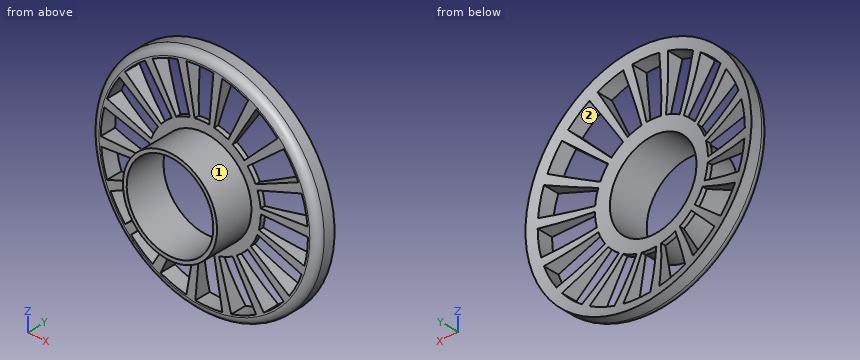
```python
from build123d import *

# Parameters (mm, degrees)
SKETCH1_R           = 12.5
BOSS_EXTRUDE1_DEPTH = 10
SKETCH3_R           = 30
BOSS_EXTRUDE2_DEPTH = 5
DOME1_FACE_RADIUS   = 30
DOME1_HEIGHT        = 5
SKETCH8_R           = 11.5
CUT_EXTRUDE3_DEPTH  = 46
CUT_EXTRUDE4_DEPTH  = 44.588989435
FILLET2_R           = 2


with BuildPart() as part:
    # Sketch1 → Boss-Extrude1 (new body)
    with BuildSketch(Plane(origin=(0, 0, 0), x_dir=(1, 0, 0), z_dir=(0, 1, 0))):
        with Locations(Location((0, 0, 0), (0, 0, 270))):
            Circle(SKETCH1_R)
    extrude(amount=BOSS_EXTRUDE1_DEPTH)

    # Sketch3 → Boss-Extrude2 (add)
    with BuildSketch(Plane(origin=(0, 10, 0), x_dir=(1, 0, 0), z_dir=(0, 1, 0))):
        with Locations(Location((0, 0, 0), (0, 0, 270))):
            Circle(SKETCH3_R)
    extrude(amount=BOSS_EXTRUDE2_DEPTH)

    # Dome1: a dome of height H over a round flat face of radius A is a cap of a sphere of radius (A * A + H * H) / (2 * H)
    dome1_r = (DOME1_FACE_RADIUS * DOME1_FACE_RADIUS + DOME1_HEIGHT * DOME1_HEIGHT) / (2 * DOME1_HEIGHT)
    dome1_base = Plane((0, 15, 0), z_dir=(0, -1, 0))
    with Locations(dome1_base.offset(DOME1_HEIGHT - dome1_r)):
        dome1_ball = Sphere(dome1_r, mode=Mode.PRIVATE)
    add(split(dome1_ball, bisect_by=dome1_base, keep=Keep.TOP, mode=Mode.PRIVATE), mode=Mode.SUBTRACT)

    # Sketch8 → Cut-Extrude3 (cut, through all)
    with BuildSketch(Plane.XZ):
        with Locations(Location((0, 0, 0), (0, 0, 270))):
            Circle(SKETCH8_R)
    extrude(amount=-CUT_EXTRUDE3_DEPTH, mode=Mode.SUBTRACT)

    # Sketch9 → Cut-Extrude4 (cut, through all)
    with BuildSketch(Plane.XZ.offset(-10)):
        with BuildLine():
            Line((-15, 0), (-27.5, 0))
            ThreePointArc((-27.5, 0), (-27.264733688, 3.589470286), (-26.562960223, 7.11752374))
            Line((-26.562960223, 7.11752374), (-14.488887394, 3.882285677))
            ThreePointArc((-14.488887394, 3.882285677), (-14.871672921, 1.957892883), (-15, 0))
        make_face()
        with BuildLine():
            Line((-12.287280664, 8.603646545), (-22.526681218, 15.773352))
            ThreePointArc((-22.526681218, 15.773352), (-24.392797912, 12.698086864), (-25.841547072, 9.405553941))
            Line((-25.841547072, 9.405553941), (-14.095389312, 5.13030215))
            ThreePointArc((-14.095389312, 5.13030215), (-13.305162498, 6.926229199), (-12.287280664, 8.603646545))
        make_face()
        with BuildLine():
            Line((-8.603646545, 12.287280664), (-15.773352, 22.526681218))
            ThreePointArc((-15.773352, 22.526681218), (-18.578730709, 20.275126762), (-21.066222186, 17.676659266))
            Line((-21.066222186, 17.676659266), (-11.490666647, 9.641814145))
            ThreePointArc((-11.490666647, 9.641814145), (-10.133853114, 11.059160052), (-8.603646545, 12.287280664))
        make_face()
        with BuildLine():
            Line((-3.882285677, 14.488887394), (-7.11752374, 26.562960223))
            ThreePointArc((-7.11752374, 26.562960223), (-10.52379439, 25.406687144), (-13.75, 23.815698604))
            Line((-13.75, 23.815698604), (-7.5, 12.990381057))
            ThreePointArc((-7.5, 12.990381057), (-5.740251485, 13.858192988), (-3.882285677, 14.488887394))
        make_face()
        with BuildLine():
            Line((1.307336141, 14.942920471), (2.396782926, 27.395354198))
            ThreePointArc((2.396782926, 27.395354198), (-1.199533153, 27.473826094), (-4.775324886, 27.082213208))
            Line((-4.775324886, 27.082213208), (-2.604722665, 14.772116295))
            ThreePointArc((-2.604722665, 14.772116295), (-0.65429081, 14.985723324), (1.307336141, 14.942920471))
        make_face()
        with BuildLine():
            Line((6.339273926, 13.594616806), (11.622002198, 24.923464144))
            ThreePointArc((11.622002198, 24.923464144), (8.269409486, 26.227216146), (4.775324886, 27.082213208))
            Line((4.775324886, 27.082213208), (2.604722665, 14.772116295))
            ThreePointArc((2.604722665, 14.772116295), (4.510586993, 14.305754261), (6.339273926, 13.594616806))
        make_face()
        with BuildLine():
            Line((10.606601718, 10.606601718), (19.445436483, 19.445436483))
            ThreePointArc((19.445436483, 19.445436483), (16.740939298, 21.817216858), (13.75, 23.815698604))
            Line((13.75, 23.815698604), (7.5, 12.990381057))
            ThreePointArc((7.5, 12.990381057), (9.131421435, 11.900300104), (10.606601718, 10.606601718))
        make_face()
        with BuildLine():
            Line((13.594616806, 6.339273926), (24.923464144, 11.622002198))
            ThreePointArc((24.923464144, 11.622002198), (23.19326476, 14.77573923), (21.066222186, 17.676659266))
            Line((21.066222186, 17.676659266), (11.490666647, 9.641814145))
            ThreePointArc((11.490666647, 9.641814145), (12.650871687, 8.059494125), (13.594616806, 6.339273926))
        make_face()
        with BuildLine():
            Line((14.942920471, 1.307336141), (27.395354198, 2.396782926))
            ThreePointArc((27.395354198, 2.396782926), (26.848140196, 5.952089383), (25.841547072, 9.405553941))
            Line((25.841547072, 9.405553941), (14.095389312, 5.13030215))
            ThreePointArc((14.095389312, 5.13030215), (14.644440107, 3.246594209), (14.942920471, 1.307336141))
        make_face()
        with BuildLine():
            Line((14.488887394, -3.882285677), (26.562960223, -7.11752374))
            ThreePointArc((26.562960223, -7.11752374), (27.264733688, -3.589470286), (27.5, 0))
            Line((27.5, 0), (15, 0))
            ThreePointArc((15, 0), (14.871672921, -1.957892883), (14.488887394, -3.882285677))
        make_face()
        with BuildLine():
            Line((12.287280664, -8.603646545), (22.526681218, -15.773352))
            ThreePointArc((22.526681218, -15.773352), (24.392797912, -12.698086864), (25.841547072, -9.405553941))
            Line((25.841547072, -9.405553941), (14.095389312, -5.13030215))
            ThreePointArc((14.095389312, -5.13030215), (13.305162498, -6.926229199), (12.287280664, -8.603646545))
        make_face()
        with BuildLine():
            Line((8.603646545, -12.287280664), (15.773352, -22.526681218))
            ThreePointArc((15.773352, -22.526681218), (18.578730709, -20.275126762), (21.066222186, -17.676659266))
            Line((21.066222186, -17.676659266), (11.490666647, -9.641814145))
            ThreePointArc((11.490666647, -9.641814145), (10.133853114, -11.059160052), (8.603646545, -12.287280664))
        make_face()
        with BuildLine():
            Line((3.882285677, -14.488887394), (7.11752374, -26.562960223))
            ThreePointArc((7.11752374, -26.562960223), (10.52379439, -25.406687144), (13.75, -23.815698604))
            Line((13.75, -23.815698604), (7.5, -12.990381057))
            ThreePointArc((7.5, -12.990381057), (5.740251485, -13.858192988), (3.882285677, -14.488887394))
        make_face()
        with BuildLine():
            Line((-1.307336141, -14.942920471), (-2.396782926, -27.395354198))
            ThreePointArc((-2.396782926, -27.395354198), (1.199533153, -27.473826094), (4.775324886, -27.082213208))
            Line((4.775324886, -27.082213208), (2.604722665, -14.772116295))
            ThreePointArc((2.604722665, -14.772116295), (0.65429081, -14.985723324), (-1.307336141, -14.942920471))
        make_face()
        with BuildLine():
            Line((-6.339273926, -13.594616806), (-11.622002198, -24.923464144))
            ThreePointArc((-11.622002198, -24.923464144), (-8.269409486, -26.227216146), (-4.775324886, -27.082213208))
            Line((-4.775324886, -27.082213208), (-2.604722665, -14.772116295))
            ThreePointArc((-2.604722665, -14.772116295), (-4.510586993, -14.305754261), (-6.339273926, -13.594616806))
        make_face()
        with BuildLine():
            Line((-10.606601718, -10.606601718), (-19.445436483, -19.445436483))
            ThreePointArc((-19.445436483, -19.445436483), (-16.740939298, -21.817216858), (-13.75, -23.815698604))
            Line((-13.75, -23.815698604), (-7.5, -12.990381057))
            ThreePointArc((-7.5, -12.990381057), (-9.131421435, -11.900300104), (-10.606601718, -10.606601718))
        make_face()
        with BuildLine():
            Line((-13.594616806, -6.339273926), (-24.923464144, -11.622002198))
            ThreePointArc((-24.923464144, -11.622002198), (-23.19326476, -14.77573923), (-21.066222186, -17.676659266))
            Line((-21.066222186, -17.676659266), (-11.490666647, -9.641814145))
            ThreePointArc((-11.490666647, -9.641814145), (-12.650871687, -8.059494125), (-13.594616806, -6.339273926))
        make_face()
        with BuildLine():
            Line((-14.942920471, -1.307336141), (-27.395354198, -2.396782926))
            ThreePointArc((-27.395354198, -2.396782926), (-26.848140196, -5.952089383), (-25.841547072, -9.405553941))
            Line((-25.841547072, -9.405553941), (-14.095389312, -5.13030215))
            ThreePointArc((-14.095389312, -5.13030215), (-14.644440107, -3.246594209), (-14.942920471, -1.307336141))
        make_face()
    extrude(amount=-CUT_EXTRUDE4_DEPTH, mode=Mode.SUBTRACT)

    # Fillet2
    fillet2_edges = [part.edges().sort_by_distance(p)[0] for p in [
        (0, 10, -30),
    ]]
    fillet(fillet2_edges, radius=FILLET2_R)


solid = part.part
```
Work out the finished part from the listing and answer in its coordinate system (mm). Face numbers are marked on the shaded views. Give positions to 0.01 mm unless a question says otherwise; leave off trailing zeros. Order: outer loops, then holes, each group sorted by start corner. A loop starts at its lowest first (then second) coordinate and runs counter-clockwise, first axis right, second up.
1. Section A-A, the plane x = 0 is taken. Determine the outline of the cut face in (y, z), and give its area (3 significant figures).
Result sheet:
outline: (0, -12.5) - (10, -12.5) - (10, -15) - (11.22, -15) arc R92.5 cw to (10.72, -11.5) - (0, -11.5) - close; (0, 11.5) - (10.72, 11.5) arc R92.5 cw to (11.22, 15) - (10, 15) - (10, 12.5) - (0, 12.5) - close; (10, -28) arc R2 ccw to (12, -30) - (15, -30) arc R92.5 cw to (14.18, -27.5) - (10, -27.5) - close; (10, 27.5) - (14.18, 27.5) arc R92.5 cw to (15, 30) - (12, 30) arc R2 ccw to (10, 28) - close
area: 47.9 mm2
2. Section B-B, the plane y = 8.5 is taken. Determine the outline of the cut face in (x, z).
Result sheet:
outline: circle Ø25 at (0, 0); hole circle Ø23 at (0, 0)
3. The mould has two halves that part along Z. Classify the marked faces 1 and 2: released by +Z, released by -Z, zero draft, split by the parting line, or undercut.
Result sheet:
face 1: split by the parting line
face 2: undercut
4. Each of these flat-tipped pins is pushed along its axis until it touches: P1, Ø5, axis at x = 15, z = 0.5, coming from the +Y side; P2, Ø2, axis at x = 17, z = -13, coming from the +Y side; P3, Ø2, axis at x = -20, y = 12.5, coming from the +Z side; P4, Ø8, axis at x = -17, y = 3, coming from the +Z side. Where does it stop, or does it pass through?
Result sheet:
P1: stops at y = 11.67
P2: stops at y = 12.75
P3: stops at z = 23.22
P4: passes through
5. Section C-C, the plane z = 16.5 is taken. Give the number of separate pieces and of enclosed holes in the cut face, and give its area (3 significant figures).
Result sheet:
separate pieces: 7
enclosed holes: 0
area: 57.8 mm2
6. Straight lines are drawn through the part: L1, parallel to X at y = 7.25, z = 0; L2, parallel to X at y = 9, z = -9; L3, parallel to X at y = 12.5, z = -20.5. For each, find the intervals that lie inside material, in ascending order.
Result sheet:
L1: x = -12.5 to -11.5, 11.5 to 12.5
L2: x = -8.67 to -7.16, 7.16 to 8.67
L3: x = -21.9 to -18.33, -11.84 to -9.56, 11.84 to 14.35, 18.33 to 21.9
